Read the model definition and answer for the solid it produces. Units are mm, in the model's axes. A direction names the side the tool comes from. Round coordinates to 2 decimals unless told otherwise and drop trailing zeros. Order: outer loops, then holes, each group sorted by start corner. A loop starts at its lowest first (then second) coordinate and runs counter-clockwise, first axis right, second up. Notation, with made-up numbers: (18.5, 14) - (38.5, 14) arc R14 ccw to (38.5, 23) - close; hole circle Ø11 at (65.5, -14). An arc over 180 degrees is marked (long way). Answer as a JSON object with one key per item and string values. Group by question number.
Q1. A cutting plane is placed at C-C on z = -3.75. Determine the outline of the cut face in (x, y), and give its area (3 significant figures).
Q2. The mould has two halves that part along Y. Classify faces 1 (the cylindrical face through (-17.55, 0.07, 0.76)), 2 (the flat face through (0, -17, 1)), 3 (the cylindrical face through (-5, 0, -2)), 4 (the cylindrical face through (8.833, -12.549, 0.76)): pulls with the +Y half, pulls with the -Y half, needs draft (parallel to the pull), parting line crosses it, or undercut.
Q3. A tool of negligible diameter and unlimited length cuts with its end or side. For faces 5 (the flat face through (-8, 8, 1.5)), 6 (the cylindrical face through (-7.167, 15.163, 0.76)), 7 (the flat face through (-4, 4, 0)), from which of +Z, -Z, +X, -X, +Y, -Y can it reach the whole face along a straight path? Write none if from no direction.
Q4. Given pin 1 Ø1 at (x, z) = (3.5, -1) entering from -Y; pin 2 Ø4 at (x, y) = (8, -13.86) entering from -Z; pin 3 Ø5 at (y, z) = (-12, -3) entering from +X; pin 4 Ø4 at (x, y) = (-16, 0) entering from +Z, each flat-ended and moving along its own axis, determine where each tip first touches the part or whether it passes through.
Q5. A cutting plane is placed at B-B on x = 0. Determine the outline of the cut face in (y, z), and give its area (3 significant figures).
Q6. Consider line 1 (Y direction, x = -8, z = 0.7); line 2 (Z direction, x = -6, y = 5.5); line 3 (Z direction, x = 11, y = -5.5). Determine where each line is inside the solid, lowest interval first.
Q7. A cutting plane is placed at A-A on y = 0. Count the separate pieces of the cut face and the enclosed holes in it, and give its area (3 significant figures).
```python
from build123d import *

# Parameters (mm, degrees)
SKETCH1_R           = 19
BOSS_EXTRUDE2_DEPTH = 1.5
SKETCH2_R           = 1.55
CUT_EXTRUDE1_DEPTH  = 6.5
SKETCH3_R           = 10.5
BOSS_EXTRUDE3_DEPTH = 3
SKETCH4_R           = 5
BOSS_EXTRUDE4_DEPTH = 5
SKETCH5_R           = 2.5
CUT_EXTRUDE2_DEPTH  = 28.207535721
CHAMFER1_SIZE       = 0.5
FILLET1_R           = 0.1


with BuildPart() as part:
    # Sketch1 → Boss-Extrude2 (new body)
    with BuildSketch(Plane.XY):
        Circle(SKETCH1_R)
    extrude(amount=BOSS_EXTRUDE2_DEPTH)

    # Sketch2 → Cut-Extrude1 (cut)
    with BuildSketch(Plane.XY.offset(1.5)):
        with BuildLine():
            ThreePointArc((8.485281374, 17), (0, 19), (-8.485281374, 17))
            Line((-8.485281374, 17), (8.485281374, 17))
        make_face()
        with BuildLine():
            Line((8.485281374, -17), (-8.485281374, -17))
            ThreePointArc((-8.485281374, -17), (0, -19), (8.485281374, -17))
        make_face()
        with Locations((-8, 13.856406461)):
            Circle(SKETCH2_R)
        with Locations((8, 13.856406461)):
            Circle(SKETCH2_R)
        with Locations((16, 0)):
            Circle(SKETCH2_R)
        with Locations((8, -13.856406461)):
            Circle(SKETCH2_R)
        with Locations((-8, -13.856406461)):
            Circle(SKETCH2_R)
        with Locations((-16, 0)):
            Circle(SKETCH2_R)
    extrude(amount=-CUT_EXTRUDE1_DEPTH, mode=Mode.SUBTRACT)

    # Sketch3 → Boss-Extrude3 (add)
    with BuildSketch(Plane.XY.offset(1.5)):
        Circle(SKETCH3_R)
    extrude(amount=BOSS_EXTRUDE3_DEPTH)

    # Sketch4 → Boss-Extrude4 (add)
    with BuildSketch(Plane(origin=(0, 0, 0), x_dir=(-1, 0, 0), z_dir=(0, 0, -1))):
        with Locations(Location((0, 0, 0), (0, 0, 180))):
            Circle(SKETCH4_R)
    extrude(amount=BOSS_EXTRUDE4_DEPTH)

    # Sketch5 → Cut-Extrude2 (cut, through all)
    with BuildSketch(Plane.XY.offset(4.5)):
        Circle(SKETCH5_R)
    extrude(amount=-CUT_EXTRUDE2_DEPTH, mode=Mode.SUBTRACT)

    # Chamfer1
    chamfer1_edges = [part.edges().sort_by_distance(p)[0] for p in [
        (-19, 0, 1.5),
        (19, 0, 1.5),
        (-10.5, 0, 4.5),
        (-5, 0, -5),
    ]]
    chamfer(chamfer1_edges, length=CHAMFER1_SIZE)

    # Fillet1
    fillet1_edges = [part.edges().sort_by_distance(p)[0] for p in [
        (-2.5, 0, -5),
        (-2.5, 0, 4.5),
    ]]
    fillet(fillet1_edges, radius=FILLET1_R)


solid = part.part
```
Result set:
{
 "1": {"outline": "circle Ø10 at (0, 0); hole circle Ø5 at (0, 0)", "area": "58.9 mm²"},
 "2": {"face 1": "undercut", "face 2": "pulls with the -Y half", "face 3": "parting line crosses it", "face 4": "undercut"},
 "3": {"face 5": "+Z", "face 6": "+Z, -Z", "face 7": "-Z"},
 "4": {"pin 1": "stops at y = -4", "pin 2": "stops at z = 0", "pin 3": "passes through", "pin 4": "stops at z = 1.5"},
 "5": {"outline": "(-17, 0) - (-5, 0) - (-5, -4.5) - (-4.5, -5) - (-2.6, -5) arc R0.1 ccw to (-2.5, -4.9) - (-2.5, 4.4) arc R0.1 ccw to (-2.6, 4.5) - (-10, 4.5) - (-10.5, 4) - (-10.5, 1.5) - (-17, 1.5) - close; (2.5, -4.9) arc R0.1 ccw to (2.6, -5) - (4.5, -5) - (5, -4.5) - (5, 0) - (17, 0) - (17, 1.5) - (10.5, 1.5) - (10.5, 4) - (10, 4.5) - (2.6, 4.5) arc R0.1 ccw to (2.5, 4.4) - close", "area": "116 mm²"},
 "6": {"line 1": "y = -17 to -15.41, -12.31 to 12.31, 15.41 to 17", "line 2": "z = 0 to 4.5", "line 3": "z = 0 to 1.5"},
 "7": {"separate pieces": "4", "enclosed holes": "0", "area": "112 mm²"}
}
